Read the model definition and answer for the solid it produces. Units are mm, in the model's axes. A direction names the side the tool comes from. Coordinates: 2 decimals unless noted, no trailing zeros. Loops run counter-clockwise (first coordinate to the right, second up) from the corner with the lowest first, then second, coordinate; pieces in that order, holes last. Notation, with made-up numbers: (74.25, 76) - (125.25, 76) arc R19 cw to (125.25, 94) - close; hole circle Ø6 at (2, 37.5). An arc over 180 degrees is marked (long way). Use CSV: the item, a comma, the result in double quotes.
```python
from build123d import *

# Parameters (mm, degrees)
SKETCH2_W           = 4
SKETCH2_H           = 8.5
BOSS_EXTRUDE1_DEPTH = 2
SKETCH3_W           = 4
SKETCH3_H           = 6
BOSS_EXTRUDE2_DEPTH = 1.6
FILLET1_R           = 1


with BuildPart() as part:
    # Sketch2 → Boss-Extrude1 (new body)
    with BuildSketch(Plane(origin=(0, 0, 0), x_dir=(1, 0, 0), z_dir=(0, 1, 0))):
        Rectangle(SKETCH2_W, SKETCH2_H)
    extrude(amount=BOSS_EXTRUDE1_DEPTH)

    # Sketch3 → Boss-Extrude2 (add)
    with BuildSketch(Plane.XZ):
        with Locations((0, -1.25)):
            Rectangle(SKETCH3_W, SKETCH3_H)
    extrude(amount=BOSS_EXTRUDE2_DEPTH)

    # Fillet1
    fillet1_edges = [part.edges().sort_by_distance(p)[0] for p in [
        (-2, -1.6, -1.25),
        (0, -1.6, -4.25),
        (2, -1.6, -1.25),
        (0, -1.6, 1.75),
    ]]
    fillet(fillet1_edges, radius=FILLET1_R)


solid = part.part
```
Q1. A tool of negligible diameter and unlimited length cuts with its end or side. For faces 1 (the face through (-1.715, -1.299, -1.208)), 2 (the face through (0, 0, 3)), from which of +Z, -Z, +X, -X, +Y, -Y can it reach the whole face along a straight path? Write none if from no direction.
Reported:
face 1,"+Z, -Z, -X, -Y"
face 2,"+Z, +X, -X, -Y"
Q2. Given P1, Ø2, axis at x = 0, z = 2.5, coming from the -Y side, flat-ended and moving along its own axis, determine where the tip first touches the part or whether it passes through.
Reported:
P1,"stops at y = -1.26"
Q3. The part is cut by section D-D on x = -1.6. Determine the outline of the cut face in (y, z).
Reported:
outline,"(-1.4, -3.85) arc R1 ccw to (-0.6, -4.25) - (2, -4.25) - (2, 4.25) - (0, 4.25) - (0, 1.75) - (-0.6, 1.75) arc R1 ccw to (-1.4, 1.35) - close"
Q4. The part is cut by section A-A on x = 0.75. Determine the outline of the cut face in (y, z).
Reported:
outline,"(-1.6, -3.25) arc R1 ccw to (-0.6, -4.25) - (2, -4.25) - (2, 4.25) - (0, 4.25) - (0, 1.75) - (-0.6, 1.75) arc R1 ccw to (-1.6, 0.75) - close"
Q5. The part is cut by section C-C on y = -0.15. Determine the outline of the cut face in (x, z).
Reported:
outline,"(-2, -4.25) - (2, -4.25) - (2, 1.75) - (-2, 1.75) - close"
Q6. The part is cut by section B-B on z = -1. Determine the outline of the cut face in (x, y), and give its area (3 significant figures).
Reported:
outline,"(-2, -0.6) arc R1 ccw to (-1, -1.6) - (1, -1.6) arc R1 ccw to (2, -0.6) - (2, 2) - (-2, 2) - close"
area,"14.0 mm²"
Q7. Find the intervals of material crossed by probe 1 along Y at (x, z) = (-1.15, 2); probe 2 along Z at (x, y) = (0, -0.25); probe 3 along X at (y, z) = (-0.8, 0.5), in increasing order. Write a range as [from, to].
Reported:
probe 1,"y = [0, 2]"
probe 2,"z = [-4.25, 1.75]"
probe 3,"x = [-1.98, 1.98]"
